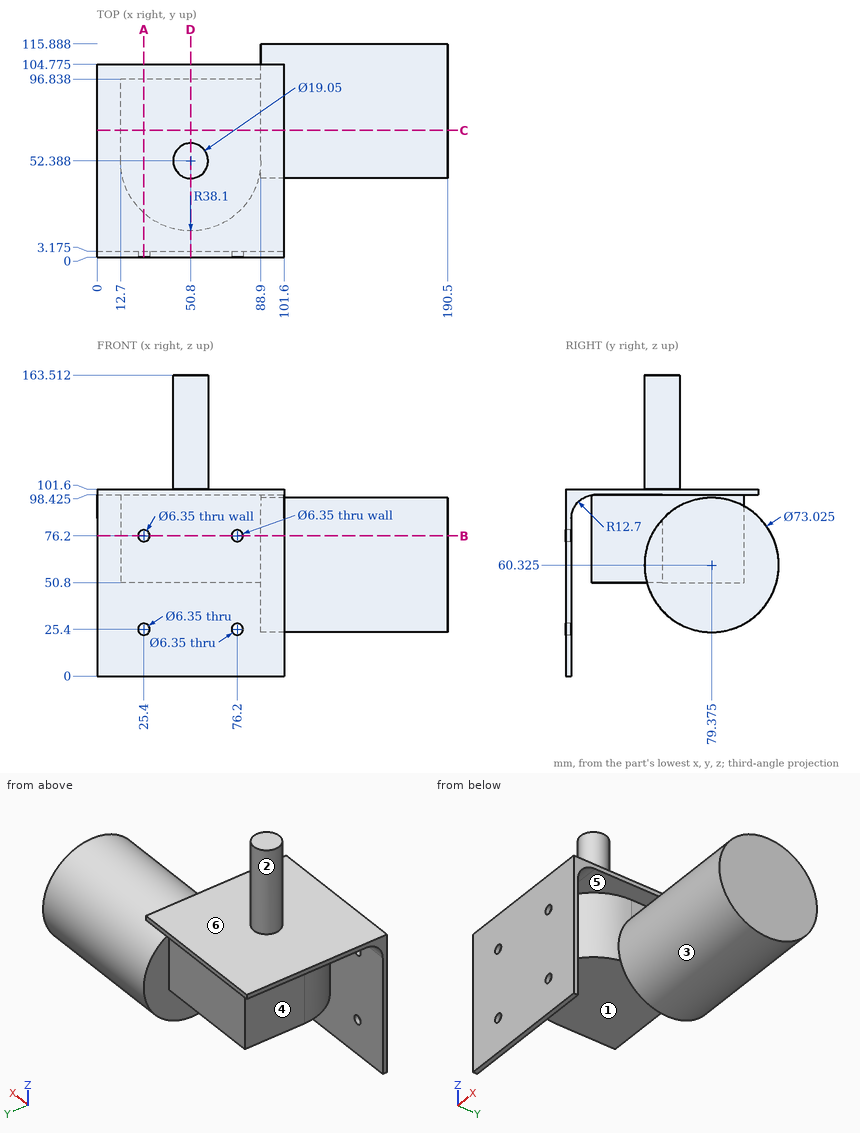
Answer from the drawing. Dimensions are ordinates in mm from the lowest x, y and z of the part. A direction names the side the tool comes from. Coordinates: 2 decimals unless noted, no trailing zeros. Loops run counter-clockwise (first coordinate to the right, second up) from the corner with the lowest first, then second, coordinate; pieces in that order, holes last. Notation, with made-up numbers: (38, 77.5) -> (70, 77.5) arc R9 ccw to (70, 81.5) -> close; hole circle Ø9 at (-22.75, 67). An arc over 180 degrees is marked (long way). Return JSON: item names as keys, results as strings.
Item 1: Find section B-B (z = 76.2). Determine the outline of the cut face in (x, y) (1 decimal).
Answers:
{"outline": "(0, 0) -> (22.2, 0) -> (22.2, 3.2) -> (0, 3.2) -> close; (12.7, 52.4) arc R38.1 ccw to (88.9, 52.4) -> (88.9, 46.5) -> (190.5, 46.5) -> (190.5, 112.3) -> (88.9, 112.3) -> (88.9, 96.8) -> (12.7, 96.8) -> close; (28.6, 0) -> (73, 0) -> (73, 3.2) -> (28.6, 3.2) -> close; (79.4, 0) -> (101.6, 0) -> (101.6, 3.2) -> (79.4, 3.2) -> close"}
Item 2: Find section C-C (y = 69). Determine the outline of the cut face in (x, z) (1 decimal), plus the area to 3 significant figures.
Answers:
{"outline": "(0, 98.4) -> (12.7, 98.4) -> (12.7, 50.8) -> (88.9, 50.8) -> (88.9, 25.3) -> (190.5, 25.3) -> (190.5, 95.3) -> (88.9, 95.3) -> (88.9, 98.4) -> (101.6, 98.4) -> (101.6, 101.6) -> (0, 101.6) -> close", "area": "11,100 mm2"}
Item 3: For a pull along Z with two mould halves and no side action, classify the marked faces 4, 5 and 6 as +Z half, -Z half, draft (parallel to the pull), parting line (faces both ways), or undercut.
Answers:
{"face 4": "draft", "face 5": "undercut", "face 6": "+Z half"}
Item 4: Find the intervals of material crossed by probe 1 along Z at (x, y) = (76, 1); probe 2 along X at (y, z) = (1, 25); probe 3 along X at (y, z) = (2.05, 76.2) (1 decimal), in increasing order.
Answers:
{"probe 1": "z = 0 to 22.23, 28.57 to 73.03, 79.37 to 101.6", "probe 2": "x = 0 to 22.25, 28.55 to 73.05, 79.35 to 101.6", "probe 3": "x = 0 to 22.2, 28.6 to 73, 79.4 to 101.6"}
Item 5: For the marked faces 1, 2 and 3, determine the directions among +Z, -Z, +X, -X, +Y, -Y from which every point of the face is accessible in a straight line to the end or side of a thin tool.
Answers:
{"face 1": "-Z, -X, +Y", "face 2": "+Z", "face 3": "+X"}
Item 6: Find section A-A (x = 25.4). Determine the outline of the cut face in (y, z) (1 decimal), plus the area to 3 significant figures.
Answers:
{"outline": "(0, 0) -> (3.2, 0) -> (3.2, 22.2) -> (0, 22.2) -> close; (0, 28.6) -> (3.2, 28.6) -> (3.2, 73) -> (0, 73) -> close; (0, 79.4) -> (3.2, 79.4) -> (3.2, 85.7) arc R12.7 cw to (15.9, 98.4) -> (24, 98.4) -> (24, 50.8) -> (96.8, 50.8) -> (96.8, 98.4) -> (104.8, 98.4) -> (104.8, 101.6) -> (0, 101.6) -> close", "area": "4,110 mm2"}
Item 7: Find section D-D (x = 50.8). Determine the outline of the cut face in (y, z) (1 decimal), plus the area to 3 significant figures.
Answers:
{"outline": "(0, 0) -> (3.2, 0) -> (3.2, 85.7) arc R12.7 cw to (14.3, 98.3) -> (14.3, 50.8) -> (96.8, 50.8) -> (96.8, 98.4) -> (104.8, 98.4) -> (104.8, 101.6) -> (61.9, 101.6) -> (61.9, 163.5) -> (42.9, 163.5) -> (42.9, 101.6) -> (0, 101.6) -> close", "area": "5,790 mm2"}
Item 8: Flat-ended cylindrical pins translate along their axes: P1, Ø22, axis at y = 64, z = 84.5, coming from the -X side; P2, Ø23, axis at x = 51, y = 55, coming from the -Z side; P3, Ø4, axis at x = 25.4, z = 76.2, coming from the -Y side. Find the tip coordinate at first contact, or state that the pin passes through.
Answers:
{"P1": "stops at x = 12.7", "P2": "stops at z = 50.8", "P3": "stops at y = 22.32"}
